Verification items for this drawing (mm, ordinates from the low corner). Round coordinates to 2 decimals unless told otherwise and drop trailing zeros. Order: outer loops, then holes, each group sorted by start corner. A loop starts at its lowest first (then second) coordinate and runs counter-clockwise, first axis right, second up. Notation, with made-up numbers: M -28.5,-33 L 27.5,-33 A24 cw 27.5,2 Z; hole C 65.5,-7 d6. An arc over 180 degrees is marked long. One line per item, written item: value. Start each with the question number.
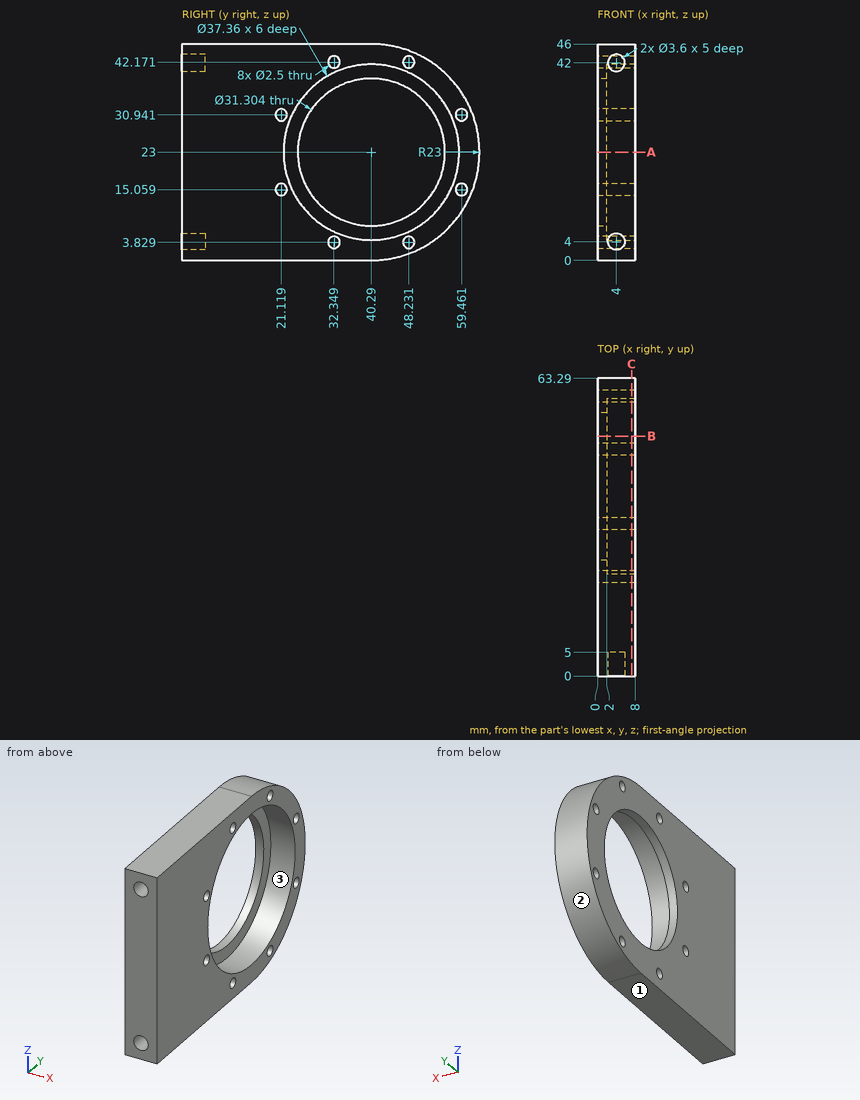
1. Draft check along Y on the marked faces 1, 2 and 3. Enter one of: released by +Y, released by -Y, zero draft, split by the parting line, or undercut.
2. Depth check by flat-ended pin: pin 1 (1.1 mm diameter, centred on x = 4.5, z = 41, fed in from -Y); pin 2 (3 mm diameter, centred on y = 32.35, z = 3.83, fed in from -X); pin 3 (5 mm diameter, centred on y = 26, z = 22, fed in from +X); pin 4 (4.5 mm diameter, centred on x = 4, z = 4, fed in from +Y). Enter the tip coordinate at first touch or a pass-through.
3. Section check B-B (y = 51). Record the cut outline in (x, z) (1 decimal).
4. Section check A-A (z = 23). Record the cut outline in (x, y).
5. Scan lines: line 1 along X through (y, z) = (1.5, 42); line 2 along Y through (x, z) = (7.5, 22.5) (1 decimal); line 3 along Y through (x, z) = (6.25, 30) (1 decimal). Record each from-to range of solid material in increasing order.
6. Section check C-C (x = 7.25). Give the number of separate pieces and of enclosed holes in the cut face, and give its area (3 significant figures).
Geometry check:
1. face 1: zero draft
1. face 2: released by +Y
1. face 3: undercut
2. pin 1: stops at y = 5
2. pin 2: stops at x = 0
2. pin 3: stops at x = 2
2. pin 4: stops at y = 56.05
3. outline: M 0,2.6 L 8,2.6 L 8,7.7 L 2,7.7 L 2,11.6 L 0,11.6 Z; M 0,34.4 L 2,34.4 L 2,38.3 L 8,38.3 L 8,43.4 L 0,43.4 Z
4. outline: M 0,0 L 8,0 L 8,21.61 L 2,21.61 L 2,24.64 L 0,24.64 Z; M 0,55.94 L 2,55.94 L 2,58.97 L 8,58.97 L 8,63.29 L 0,63.29 Z
5. line 1: x = 0 to 2.2, 5.8 to 8
5. line 2: y = 0 to 21.6, 59 to 63.3
5. line 3: y = 0 to 20.3, 21.9 to 23, 57.6 to 58.6, 60.3 to 62.2
6. separate pieces: 1
6. enclosed holes: 9
6. area: 1,550 mm²
